from build123d import *

# Parameters (mm, degrees)
SKETCH1_R           = 6.35
BOSS_EXTRUDE1_DEPTH = 6.35
SKETCH2_W           = 1.71989263
SKETCH2_H           = 1.584620177
BOSS_EXTRUDE2_DEPTH = 2.54
SKETCH3_R           = 2.499995
BOSS_EXTRUDE3_DEPTH = 38.354


with BuildPart() as part:
    # Sketch1 → Boss-Extrude1 (new body)
    with BuildSketch(Plane.XY):
        Circle(SKETCH1_R)
    extrude(amount=BOSS_EXTRUDE1_DEPTH)

    # Sketch2 → Boss-Extrude2 (add)
    with BuildSketch(Plane.XY.offset(6.35)):
        with Locations((-0.009662318, 3.043630217)):
            Rectangle(SKETCH2_W, SKETCH2_H)
    extrude(amount=BOSS_EXTRUDE2_DEPTH)

    # Sketch3 → Boss-Extrude3 (add, symmetric)
    with BuildSketch(Plane.XY.offset(6.35)):
        with Locations((0, -1.905)):
            Circle(SKETCH3_R)
    extrude(amount=BOSS_EXTRUDE3_DEPTH, both=True)


solid = part.part
Source: CAD feature listing. Evaluate the final solid. Frame: model axes, mm. A direction names the side the tool comes from. Round coordinates to 2 decimals unless told otherwise and drop trailing zeros. Loops run counter-clockwise (first coordinate to the right, second up) from the corner with the lowest first, then second, coordinate; pieces in that order, holes last. Notation, with made-up numbers: (37.25, 60) - (90.25, 60) arc R32 cw to (90.25, 94) - close; hole circle Ø11 at (70.25, 80). An arc over 180 degrees is marked (long way). Write item = value, one per line. Start each with the question number.
(1) Ray query, line 1 along Y through (x, z) = (-0.25, 6.5); line 2 along Z through (x, y) = (2.75, -2.25); line 3 along Y through (x, z) = (-2, 38) (3 decimals). Return the intervals inside material, ascending. Write a range as from..to.
(2) Section query C-C, the plane y = 5.5. Output: boundary loops of the cut face in (x, z).
(3) Pin query (flat end, axial travel): pin 1 (1.7 mm diameter, centred on x = 0, y = 2.5, fed in from +Z); pin 2 (0.5 mm diameter, centred on x = 0.5, z = 7.5, fed in from -Y); pin 3 (0.5 mm diameter, centred on x = -0.5, z = 7, fed in from +Y). Return the tip coordinate at first contact, or that it passes through.
(4) Section query A-A, the plane x = 0. Output: boundary loops of the cut face in (y, z) (3 decimals), plus the area to 3 significant figures.
(5) Section query D-D, the plane x = 3.5. Output: boundary loops of the cut face in (y, z), plus the area to 3 significant figures.
(6) Set-up query: faces 4 (the face through (-0.542, -4.346, 25.795)), 5 (the face through (0, 3, 8.89)), 6 (the face through (-0.87, 3, 8)). Return all of +Z, -Z, +X, -X, +Y, -Y with unobstructed straight access to the full face (end or side cutting, diameter ignored); none if empty.
(7) Section query B-B, the plane z = 4.5. Output: boundary loops of the cut face in (x, y), plus the area to 3 significant figures.
(8) Pull-direction query (Y, two-part tool) for faces 1 (the face through (0, 2.251, 8)), 2 (the face through (-0.542, -4.346, -15.778)), 3 (the face through (0, -2, -32.004)); classes: +Y half, -Y half, draft (parallel to the pull), parting line (faces both ways), or undercut.
Conclusion:
q1.line_1 = -4.39..0.58, 2.25..3.84
q1.line_2 = 0..6.35
q1.line_3 = -3.405..-0.405
q2.outline = (-3.17, 0) - (3.17, 0) - (3.17, 6.35) - (-3.17, 6.35) - close
q3.pin_1 = 8.89
q3.pin_2 = -4.39
q3.pin_3 = 3.84
q4.outline = (-6.35, 0) - (-4.405, 0) - (-4.405, -32.004) - (0.595, -32.004) - (0.595, 0) - (6.35, 0) - (6.35, 6.35) - (3.836, 6.35) - (3.836, 8.89) - (2.251, 8.89) - (2.251, 6.35) - (0.595, 6.35) - (0.595, 44.704) - (-4.405, 44.704) - (-4.405, 6.35) - (-6.35, 6.35) - close
q4.area = 436 mm2
q5.outline = (-5.3, 0) - (5.3, 0) - (5.3, 6.35) - (-5.3, 6.35) - close
q5.area = 67.3 mm2
q6.face_4 = +Z
q6.face_5 = +Z, +X, -X, +Y
q6.face_6 = +Z, -X, +Y
q7.outline = circle Ø12.7 at (0, 0)
q7.area = 127 mm2
q8.face_1 = undercut
q8.face_2 = parting line
q8.face_3 = draft
